Model file for the job. Use its own axes, mm. Coordinates: 2 decimals unless noted, no trailing zeros. Order: outer loops, then holes, each group sorted by start corner. A loop starts at its lowest first (then second) coordinate and runs counter-clockwise, first axis right, second up. Notation, with made-up numbers: (59, 19.25) -> (114, 19.25) arc R25 cw to (114, 41.25) -> close; hole circle Ø6 at (32.25, 52.25). An arc over 180 degrees is marked (long way). Write item = value, one per line. Start each with the question number.
Q1. Cut at B-B, the plane z = -3. List the corners of the cut face in (x, y) (3 decimals).
Q2. Flat gauge pin, fed straight in: pin 1 (1 mm diameter, centred on x = -13, y = 2, fed in from -Z). Where does the tip first touch, or does it go through?
Q3. Cut at A-A, the plane y = 4.8. List the corners of the cut face in (x, z) (3 decimals).
Q4. Wall check: line 1 (Z direction, x = -11, y = 5.25); line 2 (Y direction, x = 5.92, z = -2.5) (3 decimals); line 3 (X direction, y = 2.75, z = -3). Give the ranges that are in metal, low to high. Write a range as from..to.
Q5. Mould opens along X. For faces 1 (the face through (7.5, 1.76, -2.85)), 2 (the face through (-11.62, 4.87, -7.71)), 3 (the face through (-6, 0, -3)), 4 (the face through (11, 5, -3)) say: +X half, -X half, draft (parallel to the pull), parting line (faces both ways), or undercut.
Q6. Cut at C-C, the plane x = 5.92. List the corners of the cut face in (y, z) (3 decimals), plus the area to 3 significant figures.
Q7. Cut at D-D, the plane x = -13.5. List the corners of the cut face in (y, z).
Autodesk Inventor part; units mm, degrees
ref_plane "YZ Plane" through (0, 0, 0) normal (1, 0, 0) x (0, 1, 0)
ref_plane "XZ Plane" through (0, 0, 0) normal (0, 1, 0) x (-1, 0, 0)
ref_plane "XY Plane" through (0, 0, 0) normal (0, 0, 1) x (1, 0, 0)
sketch "Sketch1" plane through (0, 0, 0) normal (0, 1, 0) x (-1, 0, 0)
  line L0 (11, 8) -> (-11, 8)
  line L1 (-11, 8) -> (-11, -8)
  line L2 (-11, -8) -> (11, -8)
  line L3 (11, -8) -> (11, 8)
  line L4 (0, 0) -> (0, -8) construction
  line L5 (0, 0) -> (11, 0) construction
  dimension "d0" = 16
  dimension "d1" = 22
  dimension "d2" = 8
  dimension "d3" = 11
extrude "Extrusion1" add sketch "Sketch1" along normal blind 9.6
sketch "Sketch2" plane through (-11, 0, 8) normal (0, 0, 1) x (1, 0, 0)
  line L0 (22, 0) -> (22, 9.6)
  line L1 (22, 4.8) -> (16.92, 4.8) construction
  circle A0 centre (16.92, 4.8) radius 3.425
  point P0 (11, 0)
  dimension "d6" = 5.08
  dimension "d8" = 6.85
sketch "Sketch3" plane through (-11, 0, -8) normal (-1, 0, 0) x (0, 0, 1)
  point P0 (8, 0)
sketch "Sketch4" plane through (0, 9.6, 0) normal (0, 1, 0) x (1, 0, 0)
  line L0 (-11, 8) -> (-11, -8)
  line L1 (11, -8) -> (-11, -8)
  line L2 (-11, -8) -> (-11, 14)
  line L3 (-11, 14) -> (11, 14)
  line L4 (11, 14) -> (11, -8)
  point P0 (0, 0)
  dimension "d10" = 22
extrude "Extrusion2" add sketch "Sketch4" against normal blind 9.6
sketch "Sketch5" plane through (0, 9.6, 0) normal (0, 1, 0) x (1, 0, 0)
  line L0 (-11, -8) -> (-11, 14)
  circle A0 centre (-11, 3) radius 11
  point P0 (0, 0)
extrude "Extrusion3" add sketch "Sketch5" against normal blind 9.6
extrude "Extrusion4" cut sketch "Sketch2" against normal through all
sketch "Sketch6" plane through (0, 9.6, 0) normal (0, 1, 0) x (1, 0, 0)
  circle A0 centre (-11, 3) radius 6.35
  arc A1 (-11, 14) -> (-11, -8) centre (-11, 3) ccw
  point P0 (0, 0)
  dimension "d17" = 12.7
extrude "Extrusion5" cut sketch "Sketch6" against normal up to next
sketch "Sketch7" plane through (0, 9.6, 0) normal (0, 1, 0) x (1, 0, 0)
  circle A0 centre (-11, 3) radius 6.35
  circle A1 centre (-11, 3) radius 6.35
  circle A2 centre (-11, 3) radius 4.75
  point P0 (0, 0)
  dimension "d20" = 9.5
extrude "Extrusion6" add sketch "Sketch7" against normal up to surface (9.6 mm away)
equation "\"d18\" = d17"
properties part number "Bearing O"
Here are the results:
q1.outline = (-22, 0) -> (-15.75, 0) -> (-15.75, 9.6) -> (-22, 9.6) -> close; (-6.25, 0) -> (11, 0) -> (11, 9.6) -> (-6.25, 9.6) -> close; hole circle Ø6.85 at (5.92, 4.8)
q2.pin_1 = -13.9
q3.outline = (-11, -14) -> (2.495, -14) -> (2.495, 8) -> (-11, 8) arc R11 ccw to start; (9.345, -14) -> (11, -14) -> (11, 8) -> (9.345, 8) -> close; hole circle Ø9.5 at (-11, -3)
q4.line_1 = -14..-7.75, 1.75..8
q4.line_2 = 0..1.375, 8.225..9.6
q4.line_3 = -22..-15.75, -6.25..3.18, 8.66..11
q5.face_1 = undercut
q5.face_2 = undercut
q5.face_3 = draft
q5.face_4 = +X half
q6.outline = (0, -14) -> (1.375, -14) -> (1.375, 8) -> (0, 8) -> close; (8.225, -14) -> (9.6, -14) -> (9.6, 8) -> (8.225, 8) -> close
q6.area = 60.5 mm²
q7.outline = (0, -13.71) -> (9.6, -13.71) -> (9.6, -7.04) -> (0, -7.04) -> close; (0, 1.04) -> (9.6, 1.04) -> (9.6, 7.71) -> (0, 7.71) -> close
